```python
from build123d import *

# Parameters (mm, degrees)
F0_R     = 3.022598
F0_R_2   = 10.9601
F1_DEPTH = 6.35
F0_R_3   = 6.35
F2_DEPTH = 7.62


with BuildPart() as f1:
    # F0 (on Front) → F1 (new body)
    with BuildSketch(Plane.XZ):
        with BuildLine():
            Line((-6.372447, 55.266804), (50.882847, 55.266804))
            ThreePointArc((50.882847, 55.266804), (54.786488, 56.894159), (56.378253, 60.812448))
            Line((56.378253, 60.812448), (55.73595, 131.391965))
            ThreePointArc((55.73595, 131.391965), (54.108822, 135.245595), (50.240544, 136.837588))
            Line((50.240544, 136.837588), (-6.038059, 136.837588))
            ThreePointArc((-6.038059, 136.837588), (-10.764635, 134.879776), (-12.722447, 130.1532))
            Line((-12.722447, 130.1532), (-12.722447, 61.616804))
            ThreePointArc((-12.722447, 61.616804), (-10.862575, 57.126676), (-6.372447, 55.266804))
        make_face()
        with Locations((0, 76.320676)):
            Circle(F0_R, mode=Mode.SUBTRACT)
        with Locations((42.635123, 76.320676)):
            Circle(F0_R, mode=Mode.SUBTRACT)
        with Locations((21.199137, 101.73152)):
            Circle(F0_R_2, mode=Mode.SUBTRACT)
        with Locations((0, 125.187695)):
            Circle(F0_R, mode=Mode.SUBTRACT)
        with Locations((42.635123, 125.323778)):
            Circle(F0_R, mode=Mode.SUBTRACT)
    extrude(amount=F1_DEPTH)

    # F0 (on Front) → F2 (join)
    with BuildSketch(Plane.XZ):
        with Locations((21.199137, 101.73152)):
            Circle(F0_R_2)
        with Locations((21.199137, 101.73152)):
            Circle(F0_R_3, mode=Mode.SUBTRACT)
    extrude(amount=F2_DEPTH)


solid = f1.part
```
Can you work these out from the model? Positions are in its coordinate system, mm. A direction names the side the tool comes from. Round coordinates to 2 decimals unless told otherwise and drop trailing zeros. Loops run counter-clockwise (first coordinate to the right, second up) from the corner with the lowest first, then second, coordinate; pieces in that order, holes last.
Item 1: Suppose I cut it at D-D, the plane x = 8. Write out the boundary of the cut face in (y, z).
Item 2: Please list where these lines run through material, in increasing order: L1, parallel to Z at x = 0, y = -4.75; L2, parallel to Z at x = 1.5, y = -2.25; L3, parallel to X at y = -3.5, z = 79.
Item 3: Suppose I cut it at C-C, the plane x = 20. Write out the boundary of the cut face in (y, z).
Item 4: Which directions (+Z, -Z, +X, -X, +Y, -Y) give clear straight access to the entire face, cutting with the end or side of a thin tool? Please do faces 4 (the cylindrical face through (13.12, -6.98, 109.14)), 5 (the cylindrical face through (-0.393, -3.131, 128.185)).
Item 5: Suppose I cut it at A-A, the plane x = 0. Write out the boundary of the cut face in (y, z).
Item 6: If we mould it in two halves opening along X, with no side actions, what happens to faces 1 (the flat face through (22, -3, 136.838)), 2 (the cylindrical face through (24.61, -3.76, 107.09)), 3 (the flat face through (-12.722, -3, 96))? For each: +X half, -X half, draft (parallel to the pull), parting line (faces both ways), or undercut.
Item 7: Will these pins go through, and if not, where does the flat tip stop? pin 1 Ø1 at (y, z) = (-3, 96) entering from +X; pin 2 Ø5.5 at (x, z) = (42.64, 76.32) entering from +Y; pin 3 Ø10 at (x, z) = (3.5, 120.5) entering from -Y.
Item 8: Suppose I cut it at B-B, the plane y = -2.25. Write out the boundary of the cut face in (x, z), then the cut area to 3 significant figures.
Reported:
1. outline: (-6.35, 55.27) - (0, 55.27) - (0, 136.84) - (-6.35, 136.84) - close
2. L1: z = 55.27 to 73.3, 79.34 to 122.17, 128.21 to 136.84
2. L2: z = 55.27 to 73.7, 78.94 to 122.56, 127.81 to 136.84
2. L3: x = -12.72 to -1.4, 1.4 to 41.24, 44.03 to 56.21
3. outline: (-7.62, 90.84) - (-6.35, 90.84) - (-6.35, 55.27) - (0, 55.27) - (0, 95.5) - (-7.62, 95.5) - close; (-7.62, 107.97) - (0, 107.97) - (0, 136.84) - (-6.35, 136.84) - (-6.35, 112.63) - (-7.62, 112.63) - close
4. face 4: -Y
4. face 5: +Y, -Y
5. outline: (-6.35, 55.27) - (0, 55.27) - (0, 73.3) - (-6.35, 73.3) - close; (-6.35, 79.34) - (0, 79.34) - (0, 122.17) - (-6.35, 122.17) - close; (-6.35, 128.21) - (0, 128.21) - (0, 136.84) - (-6.35, 136.84) - close
6. face 1: draft
6. face 2: undercut
6. face 3: -X half
7. pin 1: stops at x = 56.06
7. pin 2: passes through
7. pin 3: stops at y = -6.35
8. outline: (-12.72, 61.62) arc R6.35 ccw to (-6.37, 55.27) - (50.88, 55.27) arc R5.5 ccw to (56.38, 60.81) - (55.74, 131.39) arc R5.5 ccw to (50.24, 136.84) - (-6.04, 136.84) arc R6.68 ccw to (-12.72, 130.15) - close; hole circle Ø6.05 at (0, 76.32); hole circle Ø6.05 at (0, 125.19); hole circle Ø12.7 at (21.2, 101.73); hole circle Ø6.05 at (42.64, 76.32); hole circle Ø6.05 at (42.64, 125.32)
8. area: 5,340 mm2
